```python
from build123d import *

# Parameters (mm, degrees)
SKETCH1_W           = 127
SKETCH1_H           = 91.44
BOSS_EXTRUDE1_DEPTH = 228.6
SKETCH3_W           = 120.65
SKETCH3_H           = 85.09
CUT_EXTRUDE1_DEPTH  = 226.06
SKETCH2_R           = 2.667
CUT_EXTRUDE2_DEPTH  = 266.475570251
SKETCH4_R           = 1.143
BOSS_EXTRUDE3_DEPTH = 5.08
SKETCH5_R           = 20.32
CUT_EXTRUDE3_DEPTH  = 1.27
FILLET1_R           = 0.762
FILLET2_R           = 0.762
FILLET3_R           = 0.762
SKETCH6_W           = 60.96
SKETCH6_H           = 25.4
CUT_EXTRUDE4_DEPTH  = 256.582569828
FILLET4_R           = 2.54
SKETCH7_W           = 85.09
SKETCH7_H           = 111.152565629
CUT_EXTRUDE5_DEPTH  = 268.942913323


with BuildPart() as part:
    # Sketch1 → Boss-Extrude1 (new body)
    with BuildSketch(Plane(origin=(0, 0, 0), x_dir=(1, 0, 0), z_dir=(0, 1, 0))):
        Rectangle(SKETCH1_W, SKETCH1_H)
    extrude(amount=BOSS_EXTRUDE1_DEPTH)

    # Sketch3 → Cut-Extrude1 (cut)
    with BuildSketch(Plane.XZ):
        Rectangle(SKETCH3_W, SKETCH3_H)
    extrude(amount=-CUT_EXTRUDE1_DEPTH, mode=Mode.SUBTRACT)

    # Sketch2 → Cut-Extrude2 (cut, through all)
    with BuildSketch(Plane(origin=(63.5, 0, 0), x_dir=(0, 0, -1), z_dir=(1, 0, 0))):
        with Locations((0, 182.88)):
            Circle(SKETCH2_R)
    extrude(amount=-CUT_EXTRUDE2_DEPTH, mode=Mode.SUBTRACT)

    # Sketch4 → Boss-Extrude3 (add)
    with BuildSketch(Plane(origin=(63.5, 0, 0), x_dir=(0, 0, -1), z_dir=(1, 0, 0))):
        with Locations(Location((-40.64, 223.52, 0), (0, 0, 180))):
            Circle(SKETCH4_R)
        with Locations(Location((40.64, 223.52, 0), (0, 0, 180))):
            Circle(SKETCH4_R)
        with Locations(Location((40.64, 142.24, 0), (0, 0, 180))):
            Circle(SKETCH4_R)
        with Locations(Location((-40.64, 142.24, 0), (0, 0, 180))):
            Circle(SKETCH4_R)
    boss_extrude3 = extrude(amount=BOSS_EXTRUDE3_DEPTH)

    # Sketch5 → Cut-Extrude3 (cut)
    with BuildSketch(Plane.ZY.offset(-60.325)):
        with Locations((0, 182.88)):
            Circle(SKETCH5_R)
    cut_extrude3 = extrude(amount=-CUT_EXTRUDE3_DEPTH, mode=Mode.SUBTRACT)

    # Fillet1
    fillet1_edges = [part.edges().sort_by_distance(p)[0] for p in [
        (61.595, 182.88, 2.667),
    ]]
    fillet(fillet1_edges, radius=FILLET1_R)

    # Fillet2
    fillet2_edges = [part.edges().sort_by_distance(p)[0] for p in [
        (63.5, 182.88, 2.667),
    ]]
    fillet(fillet2_edges, radius=FILLET2_R)

    # Mirror2: Boss-Extrude3, Cut-Extrude3 across plane
    add(boss_extrude3.mirror(Plane(origin=(0, 0, 0), x_dir=(0, 0, 1), z_dir=(1, 0, 0))))
    add(cut_extrude3.mirror(Plane(origin=(0, 0, 0), x_dir=(0, 0, 1), z_dir=(1, 0, 0))), mode=Mode.SUBTRACT)

    # Fillet3
    fillet3_edges = [part.edges().sort_by_distance(p)[0] for p in [
        (-63.5, 182.88, 2.667),
        (-61.595, 182.88, 2.667),
    ]]
    fillet(fillet3_edges, radius=FILLET3_R)

    # Sketch6 → Cut-Extrude4 (cut, through all)
    with BuildSketch(Plane.XY.offset(45.72)):
        with Locations((0, 182.88)):
            Rectangle(SKETCH6_W, SKETCH6_H)
    extrude(amount=-CUT_EXTRUDE4_DEPTH, mode=Mode.SUBTRACT)

    # Fillet4
    fillet4_edges = [part.edges().sort_by_distance(p)[0] for p in [
        (-63.5, 228.6, 0),
        (0, 228.6, 45.72),
        (63.5, 228.6, 0),
        (63.5, 114.3, 45.72),
        (-63.5, 114.3, 45.72),
        (-63.5, 114.3, -45.72),
        (63.5, 114.3, -45.72),
        (0, 228.6, -45.72),
    ]]
    fillet(fillet4_edges, radius=FILLET4_R)

    # Sketch7 → Cut-Extrude5 (cut, through all)
    with BuildSketch(Plane(origin=(63.5, 0, 0), x_dir=(0, 0, -1), z_dir=(1, 0, 0))):
        with Locations((0, 75.896282814)):
            Rectangle(SKETCH7_W, SKETCH7_H)
    extrude(amount=-CUT_EXTRUDE5_DEPTH, mode=Mode.SUBTRACT)


solid = part.part
```
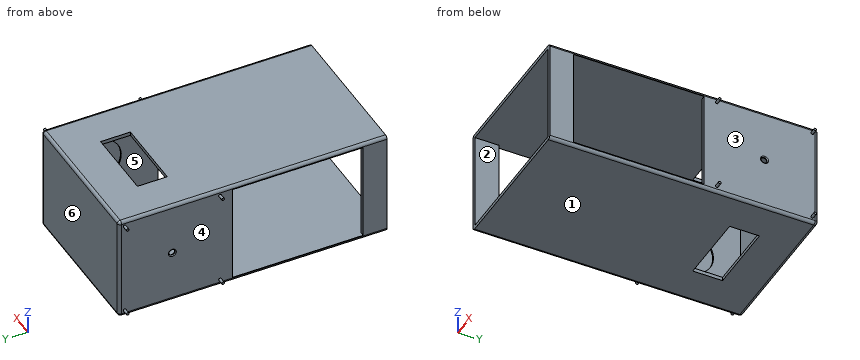
CAD build for the part. Positions are in the model's coordinates, mm. Face numbers are marked on the shaded views. A direction names the side the tool comes from. Round coordinates to 2 decimals unless told otherwise and drop trailing zeros. Order: outer loops, then holes, each group sorted by start corner. A loop starts at its lowest first (then second) coordinate and runs counter-clockwise, first axis right, second up. Notation, with made-up numbers: (9.25, -38.5) -> (19.25, -38.5) arc R24 ccw to (19.25, -1.5) -> close; hole circle Ø5 at (55.5, -14). An arc over 180 degrees is marked (long way). Write item = value, one per line.
(1) Flat gauge pins, fed straight in: P1, Ø20.5, axis at y = 182, z = 6.5, coming from the +X side; P2, Ø5, axis at x = -6.5, z = -11.5, coming from the -Y side; P3, Ø3.5, axis at y = 177, z = -44.5, coming from the -X side. Where does each tip first touch, or does it go through?
Answers follow:
P1 = 63.5
P2 = 226.06
P3 = -63.5
(2) Drill centre lines: L1, parallel to Y at x = -61, z = 0; L2, parallel to X at y = 184, z = -31 (3 decimals); L3, parallel to Z at x = 51, y = 193.5 (3 decimals). Where is each one in solid material? Low to high.
Answers follow:
L1 = 0 to 20.32, 131.47 to 162.56, 203.2 to 228.6
L2 = -63.5 to -60.325, 60.325 to 63.5
L3 = -45.72 to -42.545, 42.545 to 45.72
(3) Cut at A-A (z = -29). Write the cut outline in (x, y) (3 decimals).
Answers follow:
outline = (-63.5, 0) -> (-60.325, 0) -> (-60.325, 20.32) -> (-63.5, 20.32) -> close; (-63.5, 131.473) -> (-60.325, 131.473) -> (-60.325, 226.06) -> (60.325, 226.06) -> (60.325, 131.473) -> (63.5, 131.473) -> (63.5, 226.06) arc R2.54 ccw to (60.96, 228.6) -> (-60.96, 228.6) arc R2.54 ccw to (-63.5, 226.06) -> close; (60.325, 0) -> (63.5, 0) -> (63.5, 20.32) -> (60.325, 20.32) -> close
(4) 3-axis set-ups, long thin cutter, end or side, ignore diameter. For the marked faces 5 and 6: which of +Z, -Z, +X, -X, +Y, -Y reach the whole face in a straight line?
Answers follow:
face_5 = -Y
face_6 = +Z, -Z, +X, -X, +Y
(5) Pull direction X, two halves, no side cores. Call the marked faces 1, 2, 3 and 4: +X half, -X half, draft (parallel to the pull), parting line (faces both ways), or undercut.
Answers follow:
face_1 = draft
face_2 = undercut
face_3 = +X half
face_4 = -X half
(6) Cut at D-D (x = 42.5). Write the cut outline in (y, z) (3 decimals).
Answers follow:
outline = (0, -45.72) -> (226.06, -45.72) arc R2.54 ccw to (228.6, -43.18) -> (228.6, 43.18) arc R2.54 ccw to (226.06, 45.72) -> (0, 45.72) -> (0, 42.545) -> (226.06, 42.545) -> (226.06, -42.545) -> (0, -42.545) -> close
(7) Cut at C-C (y = 76.5). Write the cut outline in (x, z) (3 decimals).
Answers follow:
outline = (-63.5, -43.18) arc R2.54 ccw to (-60.96, -45.72) -> (60.96, -45.72) arc R2.54 ccw to (63.5, -43.18) -> (63.5, -42.545) -> (-63.5, -42.545) -> close; (-63.5, 42.545) -> (63.5, 42.545) -> (63.5, 43.18) arc R2.54 ccw to (60.96, 45.72) -> (-60.96, 45.72) arc R2.54 ccw to (-63.5, 43.18) -> close
(8) Cut at B-B (x = -6.5). Write the cut outline in (y, z) (3 decimals).
Answers follow:
outline = (0, -45.72) -> (170.18, -45.72) -> (170.18, -42.545) -> (0, -42.545) -> close; (0, 42.545) -> (170.18, 42.545) -> (170.18, 45.72) -> (0, 45.72) -> close; (195.58, -45.72) -> (226.06, -45.72) arc R2.54 ccw to (228.6, -43.18) -> (228.6, 43.18) arc R2.54 ccw to (226.06, 45.72) -> (195.58, 45.72) -> (195.58, 42.545) -> (226.06, 42.545) -> (226.06, -42.545) -> (195.58, -42.545) -> close
